Source: CAD feature listing. Evaluate the final solid. Frame: model axes, mm. Round coordinates to 2 decimals unless told otherwise and drop trailing zeros. Order: outer loops, then holes, each group sorted by start corner. A loop starts at its lowest first (then second) coordinate and runs counter-clockwise, first axis right, second up. Notation, with made-up numbers: (42, -1.75) - (68, -1.75) arc R13 cw to (68, 19.25) - close; hole circle Ø2 at (-20.75, -19). An arc over 180 degrees is marked (long way). Put each result on its own line as item: value. Start each with the question number.
1) Section D-D on z = 55. Output: boundary loops of the cut face in (x, y).
2) Section C-C on y = 20.75. Output: boundary loops of the cut face in (x, z).
3) Contact query for flat-ended pins moving along their axis: P1, Ø2.5, axis at x = 1.5, z = -54.5, coming from the -Y side; P2, Ø2.5, axis at x = 1.5, z = -51, coming from the +Y side. Output: stop coordinate, or through.
4) Section A-A on z = 31. Output: boundary loops of the cut face in (x, y).
5) Section B-B on x = 4.2. Output: boundary loops of the cut face in (y, z), then the cut area to 3 significant figures.
6) Line query: probe 1 along Y at (x, z) = (1.3, 55); probe 2 along Y at (x, z) = (3.95, -53); probe 3 along Z at (x, y) = (2.75, -5.5). Output: solid intervals per line, ascending. Write a range as [from, to].
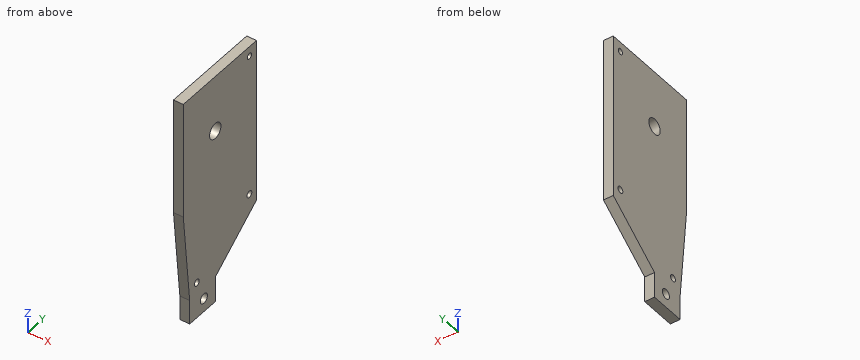
```python
from build123d import *

# Parameters (mm, degrees)
CROQUIS1_W              = 120
CROQUIS1_H              = 51.5
SALIENTE_EXTRUIR1_DEPTH = 5
CORTAR_EXTRUIR1_REACH   = 7
CORTAR_EXTRUIR2_REACH   = 7
CROQUIS3_R              = 1.5
CROQUIS3_R_2            = 4
CORTAR_EXTRUIR3_REACH   = 7
CROQUIS4_R              = 1.7
CORTAR_EXTRUIR4_REACH   = 7
CROQUIS9_R              = 2.5
CORTAR_EXTRUIR8_DEPTH   = 10


with BuildPart() as part:
    # Croquis1 → Saliente-Extruir1 (new body)
    with BuildSketch(Plane(origin=(0, 0, 0), x_dir=(0, 0, -1), z_dir=(1, 0, 0))):
        Rectangle(CROQUIS1_W, CROQUIS1_H)
    extrude(amount=SALIENTE_EXTRUIR1_DEPTH)

    # Croquis2 → Cortar-Extruir1 (cut, up to next)
    with BuildSketch(Plane(origin=(5, 0, 0), x_dir=(0, 0, -1), z_dir=(1, 0, 0)), mode=Mode.PRIVATE) as cortar_extruir1_sk1:
        Polygon((25, 25.75), (46.853067453, -3.25), (60, -3.25), (60, 25.75), align=None)
    cortar_extruir1_tool1 = extrude(cortar_extruir1_sk1.sketch, amount=-CORTAR_EXTRUIR1_REACH, mode=Mode.PRIVATE) & part.part
    add(cortar_extruir1_tool1.solids().sort_by_distance((5, 13.443767, -47.136706))[0], mode=Mode.SUBTRACT)

    # Croquis3 → Cortar-Extruir2 (cut, up to next)
    with BuildSketch(Plane(origin=(5, 0, 0), x_dir=(0, 0, -1), z_dir=(1, 0, 0)), mode=Mode.PRIVATE) as cortar_extruir2_sk1:
        with Locations((-55, 20.75)):
            Circle(CROQUIS3_R)
    cortar_extruir2_tool1 = extrude(cortar_extruir2_sk1.sketch, amount=-CORTAR_EXTRUIR2_REACH, mode=Mode.PRIVATE) & part.part
    add(cortar_extruir2_tool1.solids().sort_by_distance((5, 20.75, 55))[0], mode=Mode.SUBTRACT)
    # Croquis3 → Cortar-Extruir2 (cut, up to next)
    with BuildSketch(Plane(origin=(5, 0, 0), x_dir=(0, 0, -1), z_dir=(1, 0, 0)), mode=Mode.PRIVATE) as cortar_extruir2_sk2:
        with Locations((-31, -3.25)):
            Circle(CROQUIS3_R_2)
    cortar_extruir2_tool2 = extrude(cortar_extruir2_sk2.sketch, amount=-CORTAR_EXTRUIR2_REACH, mode=Mode.PRIVATE) & part.part
    add(cortar_extruir2_tool2.solids().sort_by_distance((5, -3.25, 31))[0], mode=Mode.SUBTRACT)

    # Croquis4 → Cortar-Extruir3 (cut, up to next)
    with BuildSketch(Plane.ZY, mode=Mode.PRIVATE) as cortar_extruir3_sk1:
        with Locations((-18.623723721, 20.75)):
            Circle(CROQUIS4_R)
    cortar_extruir3_tool1 = extrude(cortar_extruir3_sk1.sketch, amount=-CORTAR_EXTRUIR3_REACH, mode=Mode.PRIVATE) & part.part
    add(cortar_extruir3_tool1.solids().sort_by_distance((0, 20.75, -18.623724))[0], mode=Mode.SUBTRACT)
    # Croquis4 → Cortar-Extruir3 (cut, up to next)
    with BuildSketch(Plane.ZY, mode=Mode.PRIVATE) as cortar_extruir3_sk2:
        with Locations((-41.301477372, -16.25)):
            Circle(CROQUIS4_R)
    cortar_extruir3_tool2 = extrude(cortar_extruir3_sk2.sketch, amount=-CORTAR_EXTRUIR3_REACH, mode=Mode.PRIVATE) & part.part
    add(cortar_extruir3_tool2.solids().sort_by_distance((0, -16.25, -41.301477))[0], mode=Mode.SUBTRACT)

    # Croquis5 → Cortar-Extruir4 (cut, up to next)
    with BuildSketch(Plane(origin=(5, 0, 0), x_dir=(0, 0, -1), z_dir=(1, 0, 0)), mode=Mode.PRIVATE) as cortar_extruir4_sk1:
        Polygon((47.5, -21.25), (0, -25.75), (47.5, -25.75), (60, -25.75), (60, -21.25), align=None)
    cortar_extruir4_tool1 = extrude(cortar_extruir4_sk1.sketch, amount=-CORTAR_EXTRUIR4_REACH, mode=Mode.PRIVATE) & part.part
    add(cortar_extruir4_tool1.solids().sort_by_distance((5, -23.991379, -39.281609))[0], mode=Mode.SUBTRACT)

    # Croquis9 → Cortar-Extruir8 (cut)
    with BuildSketch(Plane(origin=(5, 0, 0), x_dir=(0, 0, -1), z_dir=(1, 0, 0))):
        with Locations((53, -11.25)):
            Circle(CROQUIS9_R)
    extrude(amount=-CORTAR_EXTRUIR8_DEPTH, mode=Mode.SUBTRACT)


solid = part.part
```
Answer sheet:
1. outline: (0, -25.75) - (5, -25.75) - (5, 19.25) - (0, 19.25) - close; (0, 22.25) - (5, 22.25) - (5, 25.75) - (0, 25.75) - close
2. outline: (0, -28.77) - (5, -28.77) - (5, -20.32) - (0, -20.32) - close; (0, -16.92) - (5, -16.92) - (5, 53.5) - (0, 53.5) - close; (0, 56.5) - (5, 56.5) - (5, 60) - (0, 60) - close
3. P1: y = -21.25
3. P2: y = -3.25
4. outline: (0, -25.75) - (5, -25.75) - (5, -7.25) - (0, -7.25) - close; (0, 0.75) - (5, 0.75) - (5, 25.75) - (0, 25.75) - close
5. outline: (-25.75, 0) - (-21.25, -47.5) - (-21.25, -60) - (-3.25, -60) - (-3.25, -46.85) - (25.75, -25) - (25.75, 60) - (-25.75, 60) - close; hole circle Ø3.4 at (-16.25, -41.3); hole circle Ø5 at (-11.25, -53); hole circle Ø8 at (-3.25, 31); hole circle Ø3.4 at (20.75, -18.62); hole circle Ø3 at (20.75, 55)
5. area: 5,220 mm^2
6. probe 1: [-25.75, 19.25], [22.25, 25.75]
6. probe 2: [-21.25, -13.75], [-8.75, -3.25]
6. probe 3: [-60, 27.69], [34.31, 60]
